```python
from build123d import *

# Parameters (mm, degrees)
SKETCH_1_W          = 42.7
SKETCH_1_H          = 40.6
SKETCH_1_W_2        = 36.7
SKETCH_1_H_2        = 34.6
EXTRUDE_1_DEPTH     = 50
SKETCH_2_W          = 42.7
SKETCH_2_H          = 40.6
SKETCH_2_R          = 7.5
EXTRUDE_2_DEPTH     = 4
SKETCH_3_W          = 20
SKETCH_3_H          = 40.6
EXTRUDE_3_DEPTH     = 8
SKETCH_4_R          = 2.6
CUT_EXTRUDE_1_DEPTH = 71.978253712
CUT_EXTRUDE_2_DEPTH = 4
FILLET_1_R          = 2.5
FILLET_2_R          = 1.5


with BuildPart() as part:
    # Эскиз1 → Бобышка-Вытянуть1 (new body)
    with BuildSketch(Plane.XY):
        Rectangle(SKETCH_1_W, SKETCH_1_H)
        Rectangle(SKETCH_1_W_2, SKETCH_1_H_2, mode=Mode.SUBTRACT)
    extrude(amount=EXTRUDE_1_DEPTH)

    # Эскиз2 → Бобышка-Вытянуть2 (add)
    with BuildSketch(Plane(origin=(0, 0, 0), x_dir=(-1, 0, 0), z_dir=(0, 0, -1))):
        Rectangle(SKETCH_2_W, SKETCH_2_H)
        Circle(SKETCH_2_R, mode=Mode.SUBTRACT)
    extrude(amount=EXTRUDE_2_DEPTH)

    # Эскиз3 → Бобышка-Вытянуть3 (add)
    with BuildSketch(Plane.XY.offset(50)):
        with Locations((-31.35, 0)):
            Rectangle(SKETCH_3_W, SKETCH_3_H)
    extrude_3 = extrude(amount=-EXTRUDE_3_DEPTH)

    # Эскиз4 → Вырез-Вытянуть1 (cut, through all)
    with BuildSketch(Plane.XY.offset(50)):
        with Locations((-31.35, 0)):
            Circle(SKETCH_4_R)
    cut_extrude_1 = extrude(amount=-CUT_EXTRUDE_1_DEPTH, mode=Mode.SUBTRACT)

    # Эскиз5 → Вырез-Вытянуть2 (cut)
    with BuildSketch(Plane(origin=(0, 0, 42), x_dir=(-1, 0, 0), z_dir=(0, 0, -1))):
        Polygon((36.084272207, 0), (33.717136104, 4.1), (28.982863896, 4.1), (26.615727793, 0), (28.982863896, -4.1), (33.717136104, -4.1), align=None)
    cut_extrude_2 = extrude(amount=-CUT_EXTRUDE_2_DEPTH, mode=Mode.SUBTRACT)

    # Зеркальное отражение1: Бобышка-Вытянуть3, Вырез-Вытянуть1, Вырез-Вытянуть2 across plane
    add(extrude_3.mirror(Plane(origin=(0, 0, 0), x_dir=(0, 0, 1), z_dir=(1, 0, 0))))
    add(cut_extrude_1.mirror(Plane(origin=(0, 0, 0), x_dir=(0, 0, 1), z_dir=(1, 0, 0))), mode=Mode.SUBTRACT)
    add(cut_extrude_2.mirror(Plane(origin=(0, 0, 0), x_dir=(0, 0, 1), z_dir=(1, 0, 0))), mode=Mode.SUBTRACT)

    # Скругление1
    fillet_1_edges = [part.edges().sort_by_distance(p)[0] for p in [
        (-21.35, 20.3, 19),
        (-21.35, -20.3, 19),
        (-41.35, -20.3, 46),
        (-41.35, 20.3, 46),
        (21.35, -20.3, 19),
        (21.35, 20.3, 19),
        (41.35, 20.3, 46),
        (41.35, -20.3, 46),
    ]]
    fillet(fillet_1_edges, radius=FILLET_1_R)

    # Скругление2
    fillet_2_edges = [part.edges().sort_by_distance(p)[0] for p in [
        (-18.35, 17.3, 25),
        (-18.35, -17.3, 25),
        (18.35, -17.3, 25),
        (18.35, 17.3, 25),
    ]]
    fillet(fillet_2_edges, radius=FILLET_2_R)


solid = part.part
```
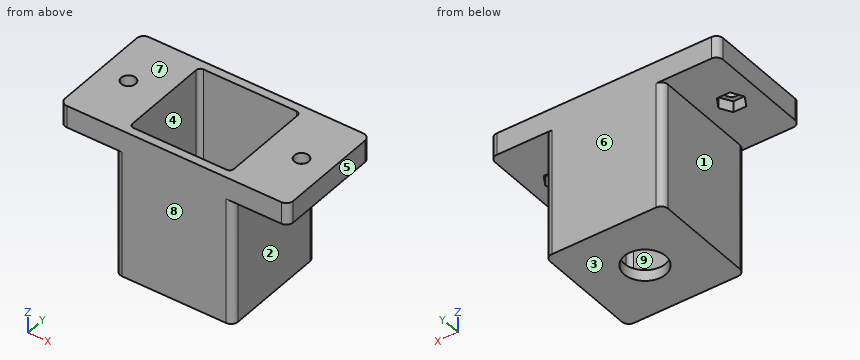
Part model, mm, in its own coordinate system. Face numbers are marked on the shaded views. A direction names the side the tool comes from. Round coordinates to 2 decimals unless told otherwise and drop trailing zeros. Order: outer loops, then holes, each group sorted by start corner. A loop starts at its lowest first (then second) coordinate and runs counter-clockwise, first axis right, second up. Notation, with made-up numbers: M 18.25,64.5 L 72.25,64.5 A30 ccw 72.25,103.5 Z; hole C -21.75,52 d6. An arc over 180 degrees is marked long. Put each result on its own line as item: value. Start each with the question number.
1. Slice it at C-C on z = 11.5. List the corners of the cut face in (x, y), then the cut area to 3 significant figures.
2. Tool access for the marked faces 1, 2, 3, 4 and 5: list every direction of +Z, -Z, +X, -X, +Y, -Y with a clear straight run to the whole face (end or side of a thin tool).
3. Slice it at B-B on x = 31.35. List the corners of the cut face in (y, z).
4. Drill centre lines: probe 1 along X at (y, z) = (-16, 9); probe 2 along X at (y, z) = (8.5, 37.5); probe 3 along Y at (x, z) = (-31.35, 48.35). Where is each one in solid material? Low to high. Write a range as [from, to].
5. Slice it at A-A on y = 6. List the corners of the cut face in (x, z).
6. Slice it at D-D on z = 43.5. List the corners of the cut face in (x, y).
7. Drop flat-ended pins along their axis: pin 1 (24 mm diameter, centred on x = 0, y = 0, fed in from -Z); pin 2 (7 mm diameter, centred on x = 32, y = 5.5, fed in from -Z); pin 3 (1 mm diameter, centred on y = -1, z = 9.5, fed in from -X); pin 4 (18 mm diameter, centred on y = -1, z = 9, fed in from +X). Give the stop position or say it passes through.
8. Two-plate mould, pull along Y, no slides. Class the marked faces 6, 7, 8 and 9: +Y half, -Y half, draft (parallel to the pull), parting line (faces both ways), or undercut.
Findings:
1. outline: M -21.35,-17.8 A2.5 ccw -18.85,-20.3 L 18.85,-20.3 A2.5 ccw 21.35,-17.8 L 21.35,17.8 A2.5 ccw 18.85,20.3 L -18.85,20.3 A2.5 ccw -21.35,17.8 Z; hole M -18.35,-15.8 A1.5 ccw -16.85,-17.3 L 16.85,-17.3 A1.5 ccw 18.35,-15.8 L 18.35,15.8 A1.5 ccw 16.85,17.3 L -16.85,17.3 A1.5 ccw -18.35,15.8 Z
1. area: 460 mm2
2. face 1: -Z, -X, +Y, -Y
2. face 2: -Z, +X, +Y, -Y
2. face 3: -Z, +X, -X, +Y, -Y
2. face 4: +Z
2. face 5: +Z, -Z, +X, +Y, -Y
3. outline: M -20.3,42 L -4.1,42 L -4.1,46 L -2.6,46 L -2.6,50 L -20.3,50 Z; M 2.6,46 L 4.1,46 L 4.1,42 L 20.3,42 L 20.3,50 L 2.6,50 Z
4. probe 1: [-21.35, -18.34], [18.34, 21.35]
4. probe 2: [-21.35, -18.35], [18.35, 21.35]
4. probe 3: [-20.3, -2.6], [2.6, 20.3]
5. outline: M -41.35,42 L -21.35,42 L -21.35,-4 L -4.5,-4 L -4.5,0 L -18.35,0 L -18.35,50 L -41.35,50 Z; M 4.5,-4 L 21.35,-4 L 21.35,42 L 41.35,42 L 41.35,50 L 18.35,50 L 18.35,0 L 4.5,0 Z
6. outline: M -41.35,-17.8 A2.5 ccw -38.85,-20.3 L 38.85,-20.3 A2.5 ccw 41.35,-17.8 L 41.35,17.8 A2.5 ccw 38.85,20.3 L -38.85,20.3 A2.5 ccw -41.35,17.8 Z; hole M -36.08,0 L -33.72,-4.1 L -28.98,-4.1 L -26.62,0 L -28.98,4.1 L -33.72,4.1 Z; hole M -18.35,-15.8 A1.5 ccw -16.85,-17.3 L 16.85,-17.3 A1.5 ccw 18.35,-15.8 L 18.35,15.8 A1.5 ccw 16.85,17.3 L -16.85,17.3 A1.5 ccw -18.35,15.8 Z; hole M 26.62,0 L 28.98,-4.1 L 33.72,-4.1 L 36.08,0 L 33.72,4.1 L 28.98,4.1 Z
7. pin 1: z = -4
7. pin 2: z = 42
7. pin 3: x = -21.35
7. pin 4: x = 21.35
8. face 6: +Y half
8. face 7: draft
8. face 8: -Y half
8. face 9: undercut
